Geometry check sheet. Reference: the model listing, model coordinates, mm. A direction names the side the tool comes from. Round coordinates to 2 decimals unless told otherwise and drop trailing zeros. Write each loop counter-clockwise with the first axis right and the second up, starting at its lowest first coordinate (ties: lowest second). Pieces come first, ordered by that corner, then holes. Notation, with made-up numbers: M -3,27 L 36,27 A28 cw 36,58 Z; hole C -19,-20.5 d8. An arc over 180 degrees is marked long. Use a Markdown table: item, result.
```python
from build123d import *

# Parameters (mm, degrees)
SKETCH1_R               = 116.84
SKETCH1_R_2             = 107.95
BOSS_EXTRUDE1_DEPTH     = 44.45
CUT_EXTRUDE6_DEPTH      = 288.798
CUT_EXTRUDE6_DEPTH_BACK = 154.94
SKETCH14_R              = 108.247485137
SKETCH15_R              = 76.2
CUT_EXTRUDE7_DEPTH      = 63.5


with BuildPart() as part:
    # Sketch1 → Boss-Extrude1 (new, symmetric)
    with BuildSketch(Plane(origin=(0, 0, 0), x_dir=(0, 0, -1), z_dir=(1, 0, 0))):
        Circle(SKETCH1_R)
        Circle(SKETCH1_R_2, mode=Mode.SUBTRACT)
    extrude(amount=BOSS_EXTRUDE1_DEPTH, both=True)

    # Sketch13 → Revolve3 (revolve)
    with BuildSketch(Plane(origin=(0, 0, 0), x_dir=(0, 0, -1), z_dir=(1, 0, 0))):
        with BuildLine():
            Line((-116.84, 0), (-116.84, -254.257018714))
            Line((-116.84, -254.257018714), (0, -254.257018714))
            Line((0, -254.257018714), (0, -116.84))
            ThreePointArc((0, -116.84), (-82.618356314, -82.618356314), (-116.84, 0))
        make_face()
    revolve(axis=Axis((0, -116.84, 0), (0, -1, 0)))

    # Sketch14 → Cut-Extrude6 (cut, two sides: drawn at the far end of the back side and taken through both)
    with BuildSketch(Plane(origin=(0, 0, 0), x_dir=(0, 0, -1), z_dir=(1, 0, 0)).offset(-CUT_EXTRUDE6_DEPTH_BACK)):
        with Locations(Location((0, 0, 0), (0, 0, 356.57852909))):
            Circle(SKETCH14_R)
    extrude(amount=CUT_EXTRUDE6_DEPTH + CUT_EXTRUDE6_DEPTH_BACK, mode=Mode.SUBTRACT)

    # Sketch15 → Cut-Extrude7 (cut)
    with BuildSketch(Plane.XZ.offset(254.257018714)):
        with Locations(Location((0, 0, 0), (0, 0, 270))):
            Circle(SKETCH15_R)
    extrude(amount=-CUT_EXTRUDE7_DEPTH, mode=Mode.SUBTRACT)


solid = part.part
```
Item 1: Cross-section at C-C, the plane x = 27.5. Record the cut outline in (y, z), and give its area (3 significant figures).
Outcome:
| item | result |
|---|---|
| outline | M -254.26,-113.56 L -27.5,-113.56 A116.84 ccw long -27.5,113.56 L -254.26,113.56 L -254.26,71.06 L -190.76,71.06 L -190.76,-71.06 L -254.26,-71.06 Z; hole C 0,0 d216.49 |
| area | 33,500 mm2 |
Item 2: Material ranges on line 1 along X through (y, z) = (-209, 0); line 2 along Y through (x, z) = (-46.5, 0); line 3 along X through (y, z) = (-121, -4.5), recorded low to high. Write a range as from..to.
Outcome:
| item | result |
|---|---|
| line 1 | x = -116.84..-76.2, 76.2..116.84 |
| line 2 | y = -190.76..-108.25 |
| line 3 | x = -116.75..116.75 |
Item 3: Cross-section at B-B, the plane y = 22. Record the cut outline in (x, z), and give its area (3 significant figures).
Outcome:
| item | result |
|---|---|
| outline | M -44.45,-114.75 L 44.45,-114.75 L 44.45,-105.99 L -44.45,-105.99 Z; M -44.45,105.99 L 44.45,105.99 L 44.45,114.75 L -44.45,114.75 Z |
| area | 1,560 mm2 |
Item 4: Go/stop test with flat-tipped pins: pin 1 (2 mm diameter, centred on x = -68.5, z = -21.5, fed in from +Y); pin 2 (1.5 mm diameter, centred on y = -110.5, z = -84, fed in from +X); pin 3 (8 mm diameter, centred on x = 39.5, z = -38, fed in from +Y). Record where each tip stops, or that it passes through.
Outcome:
| item | result |
|---|---|
| pin 1 | stops at y = -105.88 |
| pin 2 | stops at x = 81.98 |
| pin 3 | stops at y = 111.78 |
Item 5: Cross-section at D-D, the plane y = -213. Record the cut outline in (x, z).
Outcome:
| item | result |
|---|---|
| outline | C 0,0 d233.68; hole C 0,0 d152.4 |
Item 6: Access from +Z, -Z, +X, -X, +Y, -Y to the whole of each face (thin tool, end or side, straight path). Record for faces 4 (the face through (-46.367, -222.952, 60.47)), 5 (the face through (-1.636, -104.085, 29.731)).
Outcome:
| item | result |
|---|---|
| face 4 | -Y |
| face 5 | +X, -X |
Item 7: Mould release check, pull along Z, two halves, no side actions. Record for faces 1 (the face through (0.622, 116.796, -3.207)), 2 (the face through (1, -190.757, 1)), 3 (the face through (76, -254.257, 24)): +Z half, -Z half, draft (parallel to the pull), parting line (faces both ways), or undercut.
Outcome:
| item | result |
|---|---|
| face 1 | parting line |
| face 2 | undercut |
| face 3 | draft |
Item 8: Cross-section at A-A, the plane z = 0. Record the cut outline in (x, y), and give its area (3 significant figures).
Outcome:
| item | result |
|---|---|
| outline | M -116.84,-254.26 L -76.2,-254.26 L -76.2,-190.76 L 76.2,-190.76 L 76.2,-254.26 L 116.84,-254.26 L 116.84,-108.25 L -116.84,-108.25 Z; M -44.45,108.25 L 44.45,108.25 L 44.45,116.84 L -44.45,116.84 Z |
| area | 25,200 mm2 |
